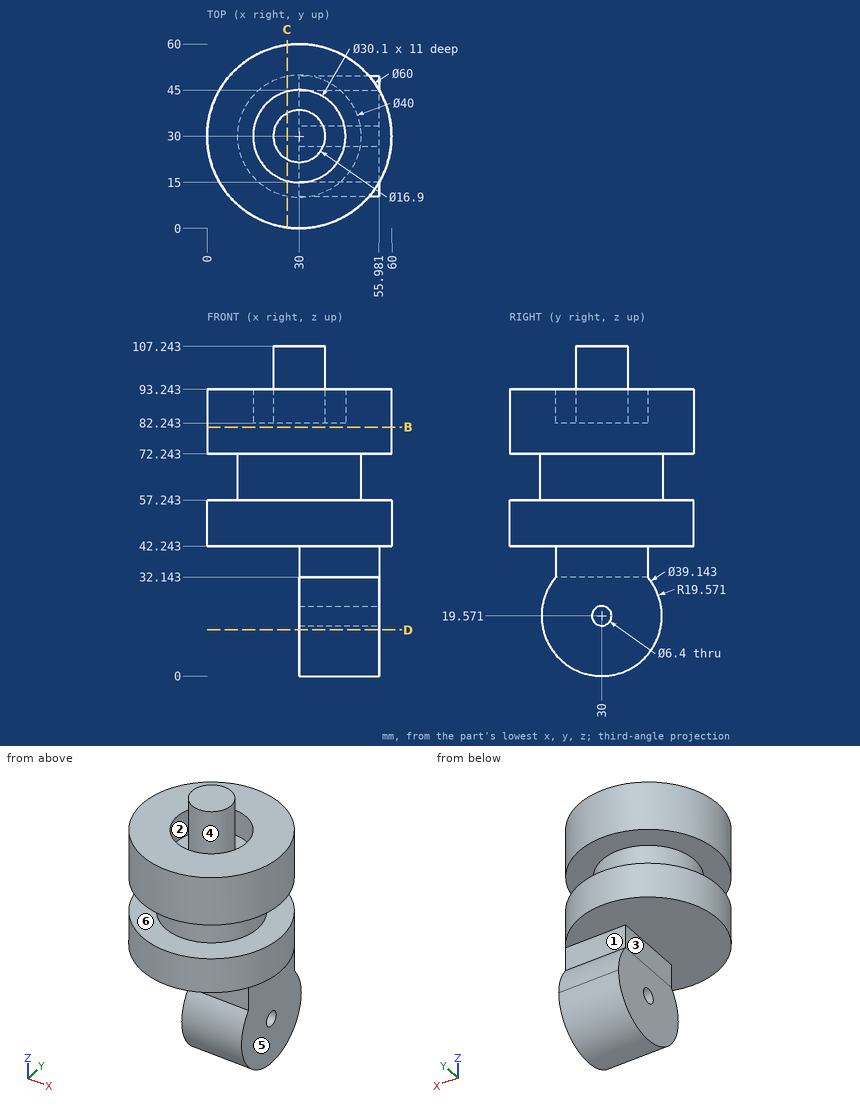
Verification items for this drawing (mm, ordinates from the low corner). A direction names the side the tool comes from. Coordinates: 2 decimals unless noted, no trailing zeros. Order: outer loops, then holes, each group sorted by start corner. A loop starts at its lowest first (then second) coordinate and runs counter-clockwise, first axis right, second up. Notation, with made-up numbers: (85, -4.75) -> (100, -4.75) arc R25 ccw to (100, 18.25) -> close; hole circle Ø2 at (82.25, 40.5). An arc over 180 degrees is marked (long way). Answer as CSV lines item,"result". Start each with the question number.
1) Material ranges on L1, parallel to Y at x = 30, z = 85.25; L2, parallel to Z at x = 43, y = 54.5; L3, parallel to Z at x = 38, y = 30, recorded low to high. Write a range as [from, to].
2) Cross-section at B-B, the plane z = 81. Record the boundary of the cut face in (x, y), then the cut area to 3 significant figures.
3) Gauge pin test, flat ends, axial feed: pin 1 Ø3 at (x, z) = (46, 38) entering from -Y; pin 2 Ø3 at (x, z) = (18.5, 55.5) entering from +Y (1 decimal); pin 3 Ø4 at (x, y) = (13, 26.5) entering from -Z. Record the tip position at first contact, or that the pin passes through.
4) Set-up check for the marked faces 4, 5 and 6: record each of +Z, -Z, +X, -X, +Y, -Y from which the full face is reachable in a straight line by a thin tool's end or side.
5) Release check for a two-part mould opening along X. For the marked faces 1, 2 and 3 record: released by +X, released by -X, zero draft, split by the parting line, or undercut.
6) Cross-section at D-D, the plane z = 15. Record the boundary of the cut face in (x, y), then the cut area to 3 significant figures.
7) Cross-section at C-C, the plane x = 26. Record the boundary of the cut face in (y, z), then the cut area to 3 significant figures.
Conclusion:
1,L1,"y = [0, 14.95], [21.55, 38.45], [45.05, 60]"
1,L2,"z = [42.24, 57.24], [72.24, 93.24]"
1,L3,"z = [0, 16.37], [22.77, 107.24]"
2,outline,"circle Ø60 at (30, 30)"
2,area,"2,830 mm²"
3,pin 1,"stops at y = 15"
3,pin 2,"stops at y = 58.3"
3,pin 3,"stops at z = 42.24"
4,face 4,"+Z"
4,face 5,"-Z, +X, +Y, -Y"
4,face 6,"none"
5,face 1,"zero draft"
5,face 2,"undercut"
5,face 3,"released by -X"
6,outline,"(30, 10.97) -> (55.98, 10.97) -> (55.98, 49.03) -> (30, 49.03) -> close"
6,area,"989 mm²"
7,outline,"(0.27, 42.24) -> (59.73, 42.24) -> (59.73, 57.24) -> (49.6, 57.24) -> (49.6, 72.24) -> (59.73, 72.24) -> (59.73, 93.24) -> (44.51, 93.24) -> (44.51, 82.24) -> (37.44, 82.24) -> (37.44, 107.24) -> (22.56, 107.24) -> (22.56, 82.24) -> (15.49, 82.24) -> (15.49, 93.24) -> (0.27, 93.24) -> (0.27, 72.24) -> (10.4, 72.24) -> (10.4, 57.24) -> (0.27, 57.24) -> close"
7,area,"2,780 mm²"
